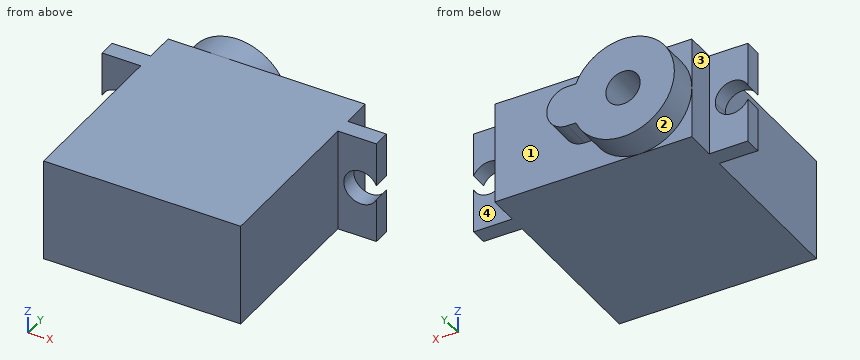
from build123d import *

# Parameters (mm, degrees)
SKETCH1_R           = 6
SKETCH1_R_2         = 2
BOSS_EXTRUDE1_DEPTH = 25
BOSS_EXTRUDE2_START = 19.5
BOSS_EXTRUDE2_DEPTH = 2
BOSS_EXTRUDE3_START = 25
SKETCH1_6_R         = 6
SKETCH1_6_R_2       = 2
BOSS_EXTRUDE3_DEPTH = 3.5
SKETCH1_7_R         = 2
BOSS_EXTRUDE4_DEPTH = 5


with BuildPart() as part:
    # Sketch1 → Boss-Extrude1 (new body)
    with BuildSketch(Plane(origin=(0, 0, 0), x_dir=(1, 0, 0), z_dir=(0, 1, 0))):
        with Locations((-5.5, 0)):
            Circle(SKETCH1_R)
        with Locations(Location((-5.5, 0, 0), (0, 0, 270))):
            Circle(SKETCH1_R_2, mode=Mode.SUBTRACT)
        with BuildLine():
            ThreePointArc((-5.499999996, 6), (-2.212713471, 5.019337334), (0, 2.397915762))
            Line((0, 2.397915762), (1, 2.397915762))
            ThreePointArc((1, 2.397915762), (3.397915762, 0), (1, -2.397915762))
            Line((1, -2.397915762), (0, -2.397915762))
            ThreePointArc((0, -2.397915762), (-2.212713472, -5.019337335), (-5.5, -6))
            Line((-5.5, -6), (11.5, -6))
            Line((11.5, -6), (11.5, 6))
            Line((11.5, 6), (-5.499999996, 6))
        make_face()
        with BuildLine():
            ThreePointArc((-5.5, -6), (-9.742640687, -4.242640687), (-11.5, 0))
            Line((-11.5, 0), (-11.5, -6))
            Line((-11.5, -6), (-5.5, -6))
        make_face()
        with BuildLine():
            Line((1, 2.397915762), (0, 2.397915762))
            ThreePointArc((0, 2.397915762), (0.373670062, 1.224744871), (0.5, 0))
            ThreePointArc((0.5, 0), (0.373670062, -1.224744871), (0, -2.397915762))
            Line((0, -2.397915762), (1, -2.397915762))
            ThreePointArc((1, -2.397915762), (3.397915762, 0), (1, 2.397915762))
        make_face()
        with BuildLine():
            ThreePointArc((-11.5, 0), (-9.742640686, 4.242640689), (-5.499999996, 6))
            Line((-5.499999996, 6), (-11.5, 6))
            Line((-11.5, 6), (-11.5, 0))
        make_face()
    extrude(amount=BOSS_EXTRUDE1_DEPTH)

    # Sketch1<4> → Boss-Extrude2 (add)
    with BuildSketch(Plane(origin=(0, 0, 0), x_dir=(1, 0, 0), z_dir=(0, 1, 0)).offset(BOSS_EXTRUDE2_START)):
        with BuildLine():
            Line((16, 6), (11.5, 6))
            Line((11.5, 6), (11.5, -6))
            Line((11.5, -6), (16, -6))
            Line((16, -6), (16, -0.871779789))
            ThreePointArc((16, -0.871779789), (12.2, 0), (16, 0.871779789))
            Line((16, 0.871779789), (16, 6))
        make_face()
        with BuildLine():
            Line((-11.5, 0), (-11.5, 6))
            Line((-11.5, 6), (-16, 6))
            Line((-16, 6), (-16, 0.871779789))
            ThreePointArc((-16, 0.871779789), (-13.752786405, 1.949358869), (-12.2, 0))
            ThreePointArc((-12.2, 0), (-13.752786405, -1.949358869), (-16, -0.871779789))
            Line((-16, -0.871779789), (-16, -6))
            Line((-16, -6), (-11.5, -6))
            Line((-11.5, -6), (-11.5, 0))
        make_face()
    extrude(amount=BOSS_EXTRUDE2_DEPTH)

    # Sketch1<6> → Boss-Extrude3 (add)
    with BuildSketch(Plane(origin=(0, 0, 0), x_dir=(1, 0, 0), z_dir=(0, 1, 0)).offset(BOSS_EXTRUDE3_START)):
        with Locations((-5.5, 0)):
            Circle(SKETCH1_6_R)
        with Locations(Location((-5.5, 0, 0), (0, 0, 270))):
            Circle(SKETCH1_6_R_2, mode=Mode.SUBTRACT)
        with BuildLine():
            Line((1, 2.397915762), (0, 2.397915762))
            ThreePointArc((0, 2.397915762), (0.373670062, 1.224744871), (0.5, 0))
            ThreePointArc((0.5, 0), (0.373670062, -1.224744871), (0, -2.397915762))
            Line((0, -2.397915762), (1, -2.397915762))
            ThreePointArc((1, -2.397915762), (3.397915762, 0), (1, 2.397915762))
        make_face()
    extrude(amount=BOSS_EXTRUDE3_DEPTH)

    # Sketch1<7> → Boss-Extrude4 (add)
    with BuildSketch(Plane(origin=(0, 0, 0), x_dir=(1, 0, 0), z_dir=(0, 1, 0))):
        with Locations(Location((-5.5, 0, 0), (0, 0, 270))):
            Circle(SKETCH1_7_R)
    extrude(amount=BOSS_EXTRUDE4_DEPTH)


solid = part.part
CAD build for the part. Positions are in the model's coordinates, mm. Face numbers are marked on the shaded views. A direction names the side the tool comes from. Give positions to 0.01 mm unless a question says otherwise; leave off trailing zeros. Loops run counter-clockwise (first coordinate to the right, second up) from the corner with the lowest first, then second, coordinate; pieces in that order, holes last. Notation, with made-up numbers: M 19,53.25 L 70,53.25 A31 cw 70,79.25 Z; hole C -21,89 d3. An arc over 180 degrees is marked long. One line per question, with ' | ' between items. Start each with the question number.
1. Saw through at D-D on z = 3.25. Give the cut face in (x, y).
2. Flat gauge pins, fed straight in: pin 1 (6 mm diameter, centred on x = 4.5, z = 2, fed in from +Y); pin 2 (1.3 mm diameter, centred on x = 13, z = 1.5, fed in from +Y); pin 3 (3 mm diameter, centred on y = 23.5, z = -2, fed in from -X); pin 4 (0.8 mm diameter, centred on x = 0.5, y = 26.5, fed in from -Z). Where does each tip first touch, or does it go through?
3. Saw through at A-A on x = 14.2. Give the cut face in (y, z).
4. Probe L1, parallel to X at y = 20.05, z = 0; L2, parallel to Z at x = 14.2, y = 20.55; L3, parallel to X at y = 1.5, z = 3.5. List the from-to ranges inside material, lowest first. Write a range as from..to.
5. Saw through at C-C on x = -2.5. Give the cut face in (y, z), plus the area to 3 significant figures.
6. 3-axis set-ups, long thin cutter, end or side, ignore diameter. For the marked faces 1, 2, 3 and 4: which of +Z, -Z, +X, -X, +Y, -Y reach the whole face in a straight line?
7. Saw through at B-B on y = 26.5. Give the cut face in (x, z), plus the area to 3 significant figures.
Result sheet:
1) outline: M -16,19.5 L -11.5,19.5 L -11.5,0 L 11.5,0 L 11.5,19.5 L 16,19.5 L 16,21.5 L 11.5,21.5 L 11.5,25 L -0.46,25 L -0.46,28.5 L -10.54,28.5 L -10.54,25 L -11.5,25 L -11.5,21.5 L -16,21.5 Z
2) pin 1: stops at y = 28.5 | pin 2: stops at y = 21.5 | pin 3: stops at x = -11.5 | pin 4: stops at z = -2.4
3) outline: M 19.5,-6 L 21.5,-6 L 21.5,-2 L 19.5,-2 Z; M 19.5,2 L 21.5,2 L 21.5,6 L 19.5,6 Z
4) L1: x = -12.2..-7.5, -3.5..12.2 | L2: z = -6..-2, 2..6 | L3: x = -11.5..11.5
5) outline: M 0,-6 L 25,-6 L 25,-5.2 L 28.5,-5.2 L 28.5,5.2 L 25,5.2 L 25,6 L 0,6 Z | area: 336 mm^2
6) face 1: +X, +Y | face 2: +Y | face 3: +Z, -Z, -X, +Y | face 4: +Z, -Z, +X, +Y
7) outline: M 0,-2.4 L 1,-2.4 A2.4 ccw 1,2.4 L 0,2.4 A6 ccw long Z; hole C -5.5,0 d4 | area: 113 mm^2
